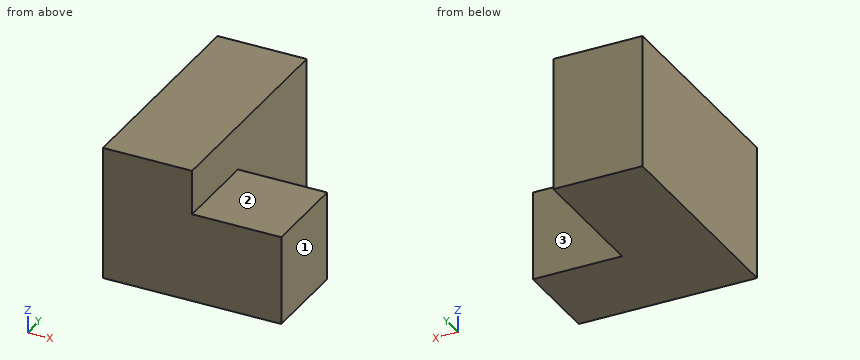
```python
from build123d import *

# Parameters (mm, degrees)
BOX001_W     = 10
BOX001_H     = 10
BOX001_DEPTH = 10
BOX_W        = 10
BOX_H        = 25
BOX_DEPTH    = 15


with BuildPart() as box001:
    # Box001 → Box001 (new body)
    with BuildSketch(Plane(origin=(10, 0, 0), x_dir=(1, 0, 0), z_dir=(0, 0, 1))):
        with Locations((5, 5)):
            Rectangle(BOX001_W, BOX001_H)
    extrude(amount=BOX001_DEPTH)


with BuildPart() as fusion001:
    # Box → Box (new body)
    with BuildSketch(Plane.XY):
        with Locations((5, 12.5)):
            Rectangle(BOX_W, BOX_H)
    extrude(amount=BOX_DEPTH)

    # Fusion: union Box001
    add(box001.part)


solid = fusion001.part
```
Verification items for the finished model (mm, model axes). Face numbers are marked on the shaded views. A direction names the side the tool comes from. Give positions to 0.01 mm unless a question says otherwise; leave off trailing zeros. Order: outer loops, then holes, each group sorted by start corner. A loop starts at its lowest first (then second) coordinate and runs counter-clockwise, first axis right, second up. Notation, with made-up numbers: M 9.25,-10.5 L 60.25,-10.5 A30 ccw 60.25,13.5 Z; hole C -24,-1.5 d6. An arc over 180 degrees is marked long. Return JSON: item names as keys, results as strings. Group by question number.
1) Section check A-A on z = 7. Record the cut outline in (x, y).
2) Section check B-B on y = 3. Record the cut outline in (x, z).
3) Go/stop test with flat-tipped pins: pin 1 Ø5 at (x, y) = (17, 5) entering from +Z; pin 2 Ø3 at (y, z) = (17.5, 6.5) entering from +X. Record where each tip stops, or that it passes through.
4) Section check D-D on z = 12.25. Record the cut outline in (x, y).
5) Access from +Z, -Z, +X, -X, +Y, -Y to the whole of each face (thin tool, end or side, straight path). Record for the marked faces 1, 2 and 3.
6) Scan line: line 1 (X direction, y = 20.75, z = 5). Record every from-to range of solid material in increasing order.
7) Section check C-C on x = 14.5. Record the cut outline in (y, z).
Answer block:
{
 "1": {"outline": "M 0,0 L 20,0 L 20,10 L 10,10 L 10,25 L 0,25 Z"},
 "2": {"outline": "M 0,0 L 20,0 L 20,10 L 10,10 L 10,15 L 0,15 Z"},
 "3": {"pin 1": "stops at z = 10", "pin 2": "stops at x = 10"},
 "4": {"outline": "M 0,0 L 10,0 L 10,25 L 0,25 Z"},
 "5": {"face 1": "+Z, -Z, +X, +Y, -Y", "face 2": "+Z, +X, +Y, -Y", "face 3": "+Z, -Z, +X, +Y"},
 "6": {"line 1": "x = 0 to 10"},
 "7": {"outline": "M 0,0 L 10,0 L 10,10 L 0,10 Z"}
}
